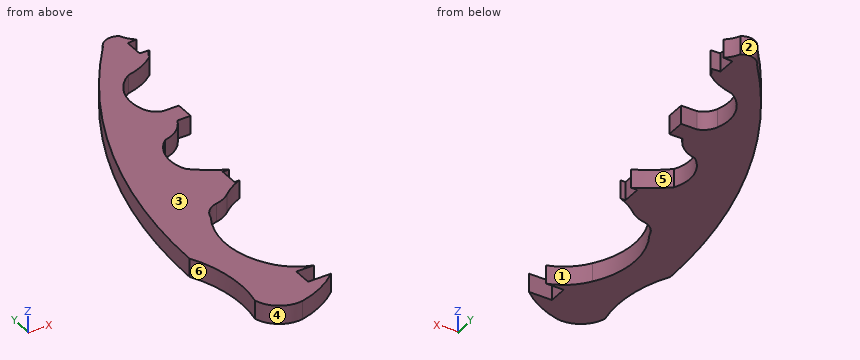
```python
from build123d import *

# Parameters (mm, degrees)
BOSS_EXTRUDE1_DEPTH = 1.524


with BuildPart() as part:
    # Sketch1 → Boss-Extrude1 (new body)
    with BuildSketch(Plane.XY):
        with BuildLine():
            Line((-110.824360774, 0), (-110.824360774, -1.524))
            Line((-110.824360774, -1.524), (-108.927743626, -1.524))
            ThreePointArc((-108.927743626, -1.524), (-110.568786986, -2.659932295), (-112.442883949, -3.346318527))
            ThreePointArc((-112.442883949, -3.346318527), (-114.17716098, -2.968961004), (-115.207793415, -1.524))
            ThreePointArc((-115.207793415, -1.524), (-115.087103351, 2.021162801), (-116.205341733, 5.387509232))
            ThreePointArc((-116.205341733, 5.387509232), (-113.752453245, 19.026762394), (-106.916865485, 31.081663004))
            ThreePointArc((-106.916865485, 31.081663004), (-106.184950927, 31.736506317), (-105.211200263, 31.608723968))
            ThreePointArc((-105.211200263, 31.608723968), (-104.901513118, 31.0579276), (-104.454303839, 30.611512291))
            Line((-104.454303839, 30.611512291), (-105.211200263, 30.544825407))
            Line((-105.211200263, 30.544825407), (-105.211200263, 29.025368505))
            Line((-105.211200263, 29.025368505), (-104.403994808, 28.977437337))
            ThreePointArc((-104.403994808, 28.977437337), (-104.700603167, 28.683060455), (-104.849681876, 28.292663471))
            ThreePointArc((-104.849681876, 28.292663471), (-106.016123504, 27.550057971), (-107.333979522, 27.131364149))
            ThreePointArc((-107.333979522, 27.131364149), (-108.818673483, 25.32832607), (-108.817338403, 22.992676119))
            ThreePointArc((-108.817338403, 22.992676119), (-108.405188947, 22.369705182), (-107.752531072, 22.00639036))
            Line((-107.752531072, 22.00639036), (-106.451038151, 22.00639036))
            Line((-106.451038151, 22.00639036), (-106.451038151, 20.478701595))
            Line((-106.451038151, 20.478701595), (-107.557691458, 20.478701595))
            ThreePointArc((-107.557691458, 20.478701595), (-108.363599409, 19.419942847), (-109.579185571, 18.87882549))
            ThreePointArc((-109.579185571, 18.87882549), (-110.645223511, 17.073742216), (-110.328866367, 15.001381081))
            ThreePointArc((-110.328866367, 15.001381081), (-109.142498989, 14.103916539), (-107.861232511, 13.348094888))
            Line((-107.861232511, 13.348094888), (-108.369232511, 13.348094888))
            Line((-108.369232511, 13.348094888), (-108.369232511, 11.811176348))
            Line((-108.369232511, 11.811176348), (-107.979675981, 11.811176348))
            ThreePointArc((-107.979675981, 11.811176348), (-108.849411149, 11.386044546), (-109.628173595, 10.810974668))
            ThreePointArc((-109.628173595, 10.810974668), (-110.216954925, 10.419220775), (-110.890927129, 10.204987173))
            ThreePointArc((-110.890927129, 10.204987173), (-111.704771273, 9.793399538), (-112.1438695, 8.994062677))
            ThreePointArc((-112.1438695, 8.994062677), (-113.066844869, 5.45696931), (-111.950245848, 1.976147619))
            ThreePointArc((-111.950245848, 1.976147619), (-110.838027473, 0.758299628), (-109.373389254, 0))
            Line((-109.373389254, 0), (-110.824360774, 0))
        make_face()
    extrude(amount=BOSS_EXTRUDE1_DEPTH)


solid = part.part
```
Can you work these out from the model? Positions are in its coordinate system, mm. Face numbers are marked on the shaded views. A direction names the side the tool comes from. Give positions to 0.01 mm unless a question says otherwise; leave off trailing zeros. Loops run counter-clockwise (first coordinate to the right, second up) from the corner with the lowest first, then second, coordinate; pieces in that order, holes last. Notation, with made-up numbers: M 62.25,-8.5 L 93.25,-8.5 A10 cw 93.25,2.5 Z; hole C -6,83.25 d11. An arc over 180 degrees is marked long. Use CSV: the item, a comma, the result in double quotes. Start each with the question number.
1. If we mould it in two halves opening along Y, with no side actions, what happens to the marked faces 3, 4, 5 and 6? For each: released by +Y, released by -Y, zero draft, split by the parting line, or undercut.
2. Imagine slicing it at B-B, the plane y = 2.5. Write out the boundary of the cut face in (x, z).
3. For P1, Ø0.5, axis at x = -109.5, z = 1, coming from the +Y side; P2, Ø0.9, axis at x = -107, z = 1, coming from the -Y side; P3, Ø0.7, axis at x = -110, z = 1, coming from the -Y side; P4, Ø1.5, axis at x = -114, y = 13.5, coming from the -Z side, each with a flat end and sliding along its axis, tell me the tip position at first contact or that it passes through.
4. If I drill on L1, parallel to Y at x = -109.25, z = 0.9; L2, parallel to X at y = 15, z = 0.2; L3, parallel to Y at x = -112, z = 0.45, over which ranges is the centre line in solid material (lowest first)?
5. On a 3-axis mill with a long thin cutter (end or side, diameter ignored), from which of +Z, -Z, +X, -X, +Y, -Y can I reach the whole of each face in a straight line? I mean the marked faces 1 and 2. Say none if no direction works.
6. Imagine slicing it at C-C, the plane x = -113.5. Write out the boundary of the cut face in (y, z).
Response values:
1,face 3,"zero draft"
1,face 4,"released by -Y"
1,face 5,"undercut"
1,face 6,"undercut"
2,outline,"M -115.17,0 L -112.27,0 L -112.27,1.52 L -115.17,1.52 Z"
3,P1,"y = 27.93"
3,P2,"y = 20.48"
3,P3,"y = -2.54"
3,P4,"z = 0"
4,L1,"-1.8 to -1.52, 11.12 to 14.18, 18.96 to 27.93"
4,L2,"-114.98 to -110.33"
4,L3,"-3.23 to 2.05, 9.4 to 23.16"
5,face 1,"+Z, -Z, +X"
5,face 2,"+Z, -Z, +Y"
6,outline,"M -3.28,0 L 19.71,0 L 19.71,1.52 L -3.28,1.52 Z"
